Input: part model. Units: mm. Frame: model coordinates. A direction names the side the tool comes from. Coordinates: 2 decimals unless noted, no trailing zeros. Loops run counter-clockwise (first coordinate to the right, second up) from the corner with the lowest first, then second, coordinate; pieces in that order, holes last. Notation, with made-up numbers: M 12.25,-39 L 56.25,-39 A16 ccw 56.25,-32 Z; hole C 72,43.5 d4. An arc over 180 degrees is marked long. Use a Markdown table: item, result. Add a question column.
1. Section B-B on y = 10. Output: boundary loops of the cut face in (x, z).
2. Draft query along X for faces 3 (the cylindrical face through (0.587, 8.874, 8.878)), 4 (the cylindrical face through (-3.977, 3.944, -6.237)), 5 (the flat face through (3, 0, 7)). Return one class per face: +X half, -X half, draft (parallel to the pull), parting line (faces both ways), or undercut.
3. Line query: L1, parallel to Z at x = 0, y = 5.75; L2, parallel to Y at x = 6, z = 1.75; L3, parallel to X at y = 7.75, z = -5.75. Output: solid intervals per line, ascending. Write a range as [from, to].
4. Pin query (flat end, axial travel): pin 1 (4 mm diameter, centred on x = 3, y = 15.5, fed in from -Z); pin 2 (1 mm diameter, centred on x = 4, y = 9.5, fed in from -Z); pin 3 (4 mm diameter, centred on x = -6.5, y = 7.5, fed in from +Z). Return the tip coordinate at first contact, or that it passes through.
5. Set-up query: faces 1 (the flat face through (0, 8, 0)), 2 (the flat face through (4, 18, 4)). Return all of +Z, -Z, +X, -X, +Y, -Y with unobstructed straight access to the full face (end or side cutting, diameter ignored); none if empty.
6. Section A-A on z = -0.5. Output: boundary loops of the cut face in (x, y), then the cut area to 3 significant figures.
Autodesk Inventor part; units mm, degrees
ref_plane "YZ Plane" through (0, 0, 0) normal (1, 0, 0) x (0, 1, 0)
ref_plane "XZ Plane" through (0, 0, 0) normal (0, 1, 0) x (-1, 0, 0)
ref_plane "XY Plane" through (0, 0, 0) normal (0, 0, 1) x (1, 0, 0)
sketch "Sketch1" plane through (0, 0, 0) normal (0, 1, 0) x (-1, 0, 0)
  point P0 (0, 0)
sketch "Sketch2" plane through (0, 0, 0) normal (0, 1, 0) x (-1, 0, 0)
  circle A0 centre (0, 0) radius 8.897
  circle A1 centre (0, 0) radius 7.397
  dimension "d0" = 17.794
  dimension "d1" = 14.794
extrude "Extrusion1" add sketch "Sketch2" along normal blind 8
sketch "Sketch3" plane through (0, 8, 0) normal (0, 1, 0) x (1, 0, 0)
  circle A0 centre (0, 0) radius 8.897
extrude "Extrusion2" add sketch "Sketch3" along normal blind 10
sketch "Sketch4" plane through (0, 18, 0) normal (0, 1, 0) x (1, 0, 0)
  arc A0 (5.25, 0) -> (-5.25, 0) centre (0, 0) ccw
  line L0 (-5.25, 0) -> (5.25, 0)
  dimension "d6" = 10.5
revolve "Revolution1" cut sketch "Sketch4" angle 360 about axis through (-5.25, 18, 0) along (-1, 0, 0)
sketch "Sketch5" plane through (0, 18, 0) normal (0, 1, 0) x (1, 0, 0)
  point P0 (0, 0)
Answers below:
| question | item | result |
|---|---|---|
| 1 | outline | C 0,0 d17.79 |
| 2 | face 3 | parting line |
| 2 | face 4 | undercut |
| 2 | face 5 | draft |
| 3 | L1 | z = [-8.9, -7.4], [7.4, 8.9] |
| 3 | L2 | y = [8, 18] |
| 3 | L3 | x = [-6.79, -4.65], [4.65, 6.79] |
| 4 | pin 1 | stops at z = -8.84 |
| 4 | pin 2 | stops at z = -8.18 |
| 4 | pin 3 | stops at z = 7.68 |
| 5 | face 1 | -Y |
| 5 | face 2 | +Z, -Z, +X, -X, +Y |
| 6 | outline | M -8.88,0 L -7.38,0 L -7.38,8 L 7.38,8 L 7.38,0 L 8.88,0 L 8.88,18 L 5.23,18 A5.23 cw -5.23,18 L -8.88,18 Z |
| 6 | area | 159 mm² |
